Can you work these out from the model? Positions are in its coordinate system, mm. A direction names the side the tool comes from. Round coordinates to 2 decimals unless told otherwise and drop trailing zeros. Write each loop counter-clockwise with the first axis right and the second up, starting at its lowest first coordinate (ties: lowest second). Pieces come first, ordered by that corner, then holes.
Q1. If we section it at C-C (x = 0.1): Please give me the cut outline in (y, z).
Q2. If we section it at D-D (z = 4.35): Please give me the cut outline in (x, y).
Q3. If we section it at A-A (z = 3.2): Please give me the cut outline in (x, y).
Q4. For faces 1 (the flat face through (-1, 2.5, 1)), 2 (the flat face through (0, 2, 3)), which set-ups out of +Z, -Z, +X, -X, +Y, -Y let a thin tool reach every point of the face, with its end or its side?
Q5. If we section it at B-B (y = -1.2): Please give me the cut outline in (x, z).
Q6. I'm going to push flat-ended pins straight in: pin 1 Ø1 at (x, y) = (1.5, 2) entering from +Z; pin 2 Ø1.5 at (x, y) = (1.5, -1.5) entering from -Z; pin 3 Ø1.6 at (x, z) = (-0.5, 4.5) entering from +Y. Where does each tip first touch, or does it pass through?
Q7. Please list where these lines run through material, in increasing order: line 1 along Y through (x, z) = (-1, 3.55); line 2 along Z through (x, y) = (2.15, 1.05); line 3 along Z through (x, y) = (-0.95, 1).
from build123d import *

# Parameters (mm, degrees)
SKETCH1_W           = 5
SKETCH1_H           = 5
BOSS_EXTRUDE1_DEPTH = 5
CUT_EXTRUDE1_DEPTH  = 4
SKETCH3_W           = 4
SKETCH3_H           = 2
CUT_EXTRUDE3_DEPTH  = 2
CUT_EXTRUDE4_DEPTH  = 2
CUT_EXTRUDE5_DEPTH  = 2
CUT_EXTRUDE6_DEPTH  = 2


with BuildPart() as part:
    # Sketch1 → Boss-Extrude1 (new body)
    with BuildSketch(Plane.XY):
        Rectangle(SKETCH1_W, SKETCH1_H)
    extrude(amount=BOSS_EXTRUDE1_DEPTH)

    # Sketch2 → Cut-Extrude1 (cut)
    with BuildSketch(Plane(origin=(2.5, 0, 0), x_dir=(0, 0, -1), z_dir=(1, 0, 0))):
        Polygon((-3, 2.5), (-5, 0.5), (-5, 2.5), align=None)
    extrude(amount=-CUT_EXTRUDE1_DEPTH, mode=Mode.SUBTRACT)

    # Sketch3 → Cut-Extrude3 (cut)
    with BuildSketch(Plane(origin=(0, 2.5, 0), x_dir=(1, 0, 0), z_dir=(0, 1, 0))):
        with Locations((0.5, -4)):
            Rectangle(SKETCH3_W, SKETCH3_H)
    extrude(amount=-CUT_EXTRUDE3_DEPTH, mode=Mode.SUBTRACT)

    # Sketch4 → Cut-Extrude4 (cut)
    with BuildSketch(Plane(origin=(2.5, 0, 0), x_dir=(0, 0, -1), z_dir=(1, 0, 0))):
        Polygon((-3, 0.5), (-5, -1.5), (-5, 0.5), align=None)
    extrude(amount=-CUT_EXTRUDE4_DEPTH, mode=Mode.SUBTRACT)

    # Sketch5 → Cut-Extrude5 (cut)
    with BuildSketch(Plane.XY.offset(3)):
        Polygon((0.5, 2.5), (2.5, 0.5), (2.5, 2.5), align=None)
    extrude(amount=-CUT_EXTRUDE5_DEPTH, mode=Mode.SUBTRACT)

    # Sketch6 → Cut-Extrude6 (cut, through all)
    with BuildSketch(Plane(origin=(-1.5, 0, 0), x_dir=(0, 0, -1), z_dir=(1, 0, 0))):
        Polygon((-3, 2.5), (-5, 0.5), (-5, 2.5), align=None)
    extrude(amount=-CUT_EXTRUDE6_DEPTH, mode=Mode.SUBTRACT)


solid = part.part
A:
1. outline: (-2.5, 0) - (2.5, 0) - (2.5, 3) - (0.5, 3) - (0.5, 5) - (-2.5, 5) - close
2. outline: (-2.5, -2.5) - (2.5, -2.5) - (2.5, -0.85) - (0.5, -0.85) - (0.5, 0.5) - (-1.5, 0.5) - (-1.5, 1.15) - (-2.5, 1.15) - close
3. outline: (-2.5, -2.5) - (2.5, -2.5) - (2.5, 0.3) - (0.5, 0.3) - (0.5, 0.5) - (-1.5, 0.5) - (-1.5, 2.3) - (-2.5, 2.3) - close
4. face 1: +Z, -Z, +X, -X, +Y
4. face 2: +Z, +X, +Y
5. outline: (-2.5, 0) - (2.5, 0) - (2.5, 4.7) - (0.5, 4.7) - (0.5, 5) - (-2.5, 5) - close
6. pin 1: stops at z = 3
6. pin 2: stops at z = 0
6. pin 3: stops at y = 0.5
7. line 1: y = -2.5 to 0.5
7. line 2: z = 0 to 1
7. line 3: z = 0 to 3
